from build123d import *

# Parameters (mm, degrees)
SKETCH1_W           = 35.56
SKETCH1_H           = 35.56
BOSS_EXTRUDE1_DEPTH = 4.5
SKETCH2_W           = 35.56
SKETCH2_H           = 35.56
BOSS_EXTRUDE2_DEPTH = 2
SKETCH5_R           = 11
BOSS_EXTRUDE5_DEPTH = 2
SKETCH6_R           = 3.175
BOSS_EXTRUDE6_DEPTH = 24
SKETCH7_R           = 2
CUT_EXTRUDE3_DEPTH  = 29
SKETCH8_W           = 31.56
SKETCH8_H           = 31.56
BOSS_EXTRUDE7_DEPTH = 25
SKETCH9_W           = 35.56
SKETCH9_H           = 35.56
BOSS_EXTRUDE8_DEPTH = 6
CHAMFER1_SIZE       = 6
SCALE1_SCALE        = 0.85
CUT_EXTRUDE4_START  = -8.5
SKETCH10_R          = 2.69875
CUT_EXTRUDE4_DEPTH  = 8.5


with BuildPart() as part:
    # Sketch1 → Boss-Extrude1 (new body)
    with BuildSketch(Plane.XY):
        with Locations((21.15, 20.624391857)):
            Rectangle(SKETCH1_W, SKETCH1_H)
    extrude(amount=BOSS_EXTRUDE1_DEPTH)

    # Sketch2 → Boss-Extrude2 (add)
    with BuildSketch(Plane.XY.offset(4.5)):
        with Locations((21.15, 20.624391857)):
            Rectangle(SKETCH2_W, SKETCH2_H)
    extrude(amount=BOSS_EXTRUDE2_DEPTH)

    # Sketch5 → Boss-Extrude5 (add)
    with BuildSketch(Plane(origin=(0, 0, 0), x_dir=(-1, 0, 0), z_dir=(0, 0, -1))):
        with Locations((-21.15, 20.624391857)):
            Circle(SKETCH5_R)
    extrude(amount=BOSS_EXTRUDE5_DEPTH)

    # Sketch6 → Boss-Extrude6 (add)
    with BuildSketch(Plane(origin=(0, 0, -2), x_dir=(-1, 0, 0), z_dir=(0, 0, -1))):
        with Locations((-21.15, 20.624391857)):
            Circle(SKETCH6_R)
    extrude(amount=BOSS_EXTRUDE6_DEPTH)

    # Sketch7 → Cut-Extrude3 (cut)
    with BuildSketch(Plane(origin=(0, 0, 0), x_dir=(-1, 0, 0), z_dir=(0, 0, -1))):
        with Locations((-35.65, 6.124391857)):
            Circle(SKETCH7_R)
        with Locations((-6.65, 6.124391857)):
            Circle(SKETCH7_R)
        with Locations((-6.65, 35.124391857)):
            Circle(SKETCH7_R)
        with Locations((-35.65, 35.124391857)):
            Circle(SKETCH7_R)
    extrude(amount=-CUT_EXTRUDE3_DEPTH, mode=Mode.SUBTRACT)

    # Sketch8 → Boss-Extrude7 (add)
    with BuildSketch(Plane.XY.offset(6.5)):
        with Locations((21.15, 20.624391857)):
            Rectangle(SKETCH8_W, SKETCH8_H)
    extrude(amount=BOSS_EXTRUDE7_DEPTH)

    # Sketch9 → Boss-Extrude8 (add)
    with BuildSketch(Plane.XY.offset(31.5)):
        with Locations((21.15, 20.624391857)):
            Rectangle(SKETCH9_W, SKETCH9_H)
    extrude(amount=BOSS_EXTRUDE8_DEPTH)

    # Chamfer1
    # the kernel refuses this chamfer: 6 mm, written as the material it takes off along each edge
    with BuildSketch(Plane(origin=(5.37, 36.404391857, 6.5), x_dir=(0.9996219169112968, 0.02749587661058678, 0), z_dir=(0, 0, 1)), Plane(origin=(36.93, 4.844391857, 6.5), x_dir=(-0.9996219169112969, -0.027495876610586355, 0), z_dir=(0, 0, 1)), Plane(origin=(36.93, 36.404391857, 6.5), x_dir=(0.02749587661058678, -0.9996219169112968, 0), z_dir=(0, 0, 1))) as chamfer1_piece_1:
        Polygon((CHAMFER1_SIZE * 0.999621916911, -CHAMFER1_SIZE * 0.0274958766106), (-CHAMFER1_SIZE * 0.0274958766106, -CHAMFER1_SIZE * 0.999621916911), (0, 0), align=None)
    extrude(amount=25, mode=Mode.SUBTRACT)
    with BuildSketch(Plane(origin=(5.37, 4.844391857, 6.5), x_dir=(0.9996219169112969, -0.027495876610586348, 0), z_dir=(0, 0, 1))) as chamfer1_piece_2:
        Polygon((CHAMFER1_SIZE * 0.999621916911, CHAMFER1_SIZE * 0.0274958766106), (-CHAMFER1_SIZE * 0.0274958766106, CHAMFER1_SIZE * 0.999621916911), (0, 0), align=None)
    extrude(amount=25, mode=Mode.SUBTRACT)


with BuildPart() as part_1:
    # Scale1: scaled about (21.15, 20.624391857, 17.82804973)
    add(part.part.scale(SCALE1_SCALE).moved(Location((3.1725, 3.093658779, 2.67420746))))

    # Sketch10 → Cut-Extrude4 (cut)
    with BuildSketch(Plane(origin=(0, 0, -19.425792541), x_dir=(-1, 0, 0), z_dir=(0, 0, -1)).offset(CUT_EXTRUDE4_START)):
        with Locations((-21.15, 20.624391857)):
            Circle(SKETCH10_R)
    extrude(amount=CUT_EXTRUDE4_DEPTH, mode=Mode.SUBTRACT)


solid = part_1.part
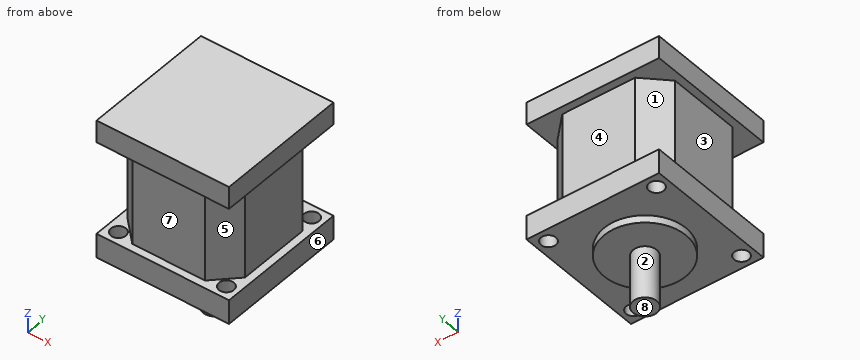
Verification items for the finished model (mm, model axes). Face numbers are marked on the shaded views. A direction names the side the tool comes from. Round coordinates to 2 decimals unless told otherwise and drop trailing zeros. Loops run counter-clockwise (first coordinate to the right, second up) from the corner with the lowest first, then second, coordinate; pieces in that order, holes last. Notation, with made-up numbers: (74.25, 23.25) - (128.25, 23.25) arc R15 cw to (128.25, 49.25) - close; hole circle Ø11 at (72, -27.5). An arc over 180 degrees is marked (long way). Use a Markdown table: item, result. Add a question column.
1. Thickness scan on probe 1 along Y at (x, z) = (9, 7); probe 2 along Z at (x, y) = (25, 34.5); probe 3 along Z at (x, y) = (31, 15). Record the ranges inside material, lowest first. Write a range as [from, to].
2. Access from +Z, -Z, +X, -X, +Y, -Y to the whole of each face (thin tool, end or side, straight path). Record for the marked faces 1, 2, 3 and 4.
3. Section check B-B, the plane z = 11. Record the boundary of the cut face in (x, y), plus the area to 3 significant figures.
4. Section check D-D, the plane y = 22.5. Record the boundary of the cut face in (x, z).
5. Section check C-C, the plane y = 16. Record the boundary of the cut face in (x, z), plus the area to 3 significant figures.
6. Release check for a two-part mould opening along Z. For the marked faces 5, 6, 7 and 8 record: released by +Z, released by -Z, zero draft, split by the parting line, or undercut.
7. Gauge pin test, flat ends, axial feed: pin 1 (4 mm diameter, centred on x = 8.82, y = 32.95, fed in from -Z); pin 2 (13.5 mm diameter, centred on x = 19.5, z = 21, fed in from +Y); pin 3 (1 mm diameter, centred on y = 31.5, z = 11, fed in from +X). Record the tip position at first contact, or that the pin passes through.
8. Section check A-A, the plane x = 21.15. Record the boundary of the cut face in (y, z), plus the area to 3 significant figures.
Checks:
| question | item | result |
|---|---|---|
| 1 | probe 1 | y = [5.51, 6.61], [9.99, 31.26], [34.64, 35.74] |
| 1 | probe 2 | z = [2.67, 8.2], [29.45, 34.55] |
| 1 | probe 3 | z = [2.67, 34.55] |
| 2 | face 1 | -X, +Y |
| 2 | face 2 | -Z |
| 2 | face 3 | -X, +Y, -Y |
| 2 | face 4 | +X, -X, +Y |
| 3 | outline | (7.74, 12.31) - (12.84, 7.21) - (29.46, 7.21) - (34.56, 12.31) - (34.56, 28.94) - (29.46, 34.04) - (12.84, 34.04) - (7.74, 28.94) - close |
| 3 | area | 668 mm^2 |
| 4 | outline | (6.04, 2.67) - (11.99, 2.67) - (11.99, 0.97) - (19.21, 0.97) - (19.21, -10.93) - (23.09, -10.93) - (23.09, 0.97) - (30.31, 0.97) - (30.31, 2.67) - (36.26, 2.67) - (36.26, 8.2) - (34.56, 8.2) - (34.56, 29.45) - (36.26, 29.45) - (36.26, 34.55) - (6.04, 34.55) - (6.04, 29.45) - (7.74, 29.45) - (7.74, 8.2) - (6.04, 8.2) - close |
| 5 | outline | (6.04, 2.67) - (13.02, 2.67) - (13.02, 0.97) - (29.28, 0.97) - (29.28, 2.67) - (36.26, 2.67) - (36.26, 8.2) - (34.56, 8.2) - (34.56, 29.45) - (36.26, 29.45) - (36.26, 34.55) - (6.04, 34.55) - (6.04, 29.45) - (7.74, 29.45) - (7.74, 8.2) - (6.04, 8.2) - close |
| 5 | area | 919 mm^2 |
| 6 | face 5 | undercut |
| 6 | face 6 | zero draft |
| 6 | face 7 | undercut |
| 6 | face 8 | released by -Z |
| 7 | pin 1 | stops at z = 2.67 |
| 7 | pin 2 | stops at y = 34.04 |
| 7 | pin 3 | stops at x = 32.5 |
| 8 | outline | (5.51, 2.67) - (11.27, 2.67) - (11.27, 0.97) - (17.93, 0.97) - (17.93, -10.93) - (23.32, -10.93) - (23.32, 0.97) - (29.97, 0.97) - (29.97, 2.67) - (35.74, 2.67) - (35.74, 8.2) - (34.04, 8.2) - (34.04, 29.45) - (35.74, 29.45) - (35.74, 34.55) - (5.51, 34.55) - (5.51, 29.45) - (7.21, 29.45) - (7.21, 8.2) - (5.51, 8.2) - close |
| 8 | area | 987 mm^2 |
